Verification items for the finished model (mm, model axes). Coordinates: 2 decimals unless noted, no trailing zeros. Order: outer loops, then holes, each group sorted by start corner. A loop starts at its lowest first (then second) coordinate and runs counter-clockwise, first axis right, second up.
Q1. Depth check by flat-ended pin: P1, Ø6.5, axis at x = -5, z = -42.5, coming from the -Y side; P2, Ø3.5, axis at x = -5, z = -30, coming from the +Y side. Enter the tip coordinate at first touch or a pass-through.
Q2. Cross-section at A-A, the plane z = -42.5. Record the boundary of the cut face in (x, y).
Q3. Thickness scan on line 1 (Z direction, x = -5, y = 0.6); line 2 (X direction, y = 2.8, z = -16); line 3 (X direction, y = 2.6, z = -31). Record the ranges inside material, lowest first.
Q4. Draft check along X on faces 1 (the flat face through (-25, 0, -30)), 2 (the cylindrical face through (-4.74, 1.479, -19.483)), 3 (the flat face through (0, 1, -30)). Enter one of: pulls with the +X half, pulls with the -X half, needs draft (parallel to the pull), parting line crosses it, or undercut.
Autodesk Inventor part; units mm, degrees
ref_plane "YZ Plane" through (0, 0, 0) normal (1, 0, 0) x (0, 1, 0)
ref_plane "XZ Plane" through (0, 0, 0) normal (0, 1, 0) x (-1, 0, 0)
ref_plane "XY Plane" through (0, 0, 0) normal (0, 0, 1) x (1, 0, 0)
sketch "Sketch1" plane through (0, 0, 0) normal (0, 1, 0) x (-1, 0, 0)
  line L0 (0, 0) -> (50, 0)
  line L1 (50, 0) -> (50, -60)
  line L2 (50, -60) -> (0, -60)
  line L3 (0, -60) -> (0, 0)
  circle A0 centre (5, -30) radius 2
  circle A1 centre (5, -42.5) radius 2
  circle A2 centre (5, -17.5) radius 2
  dimension "d0" = 50
  dimension "d1" = 60
  dimension "d2" = 4
  dimension "d3" = 4
  dimension "d4" = 4
extrude "Extrusion1" add sketch "Sketch1" along normal blind 3
properties part number "dc clamps"
Check values:
1. P1: stops at y = 0
1. P2: passes through
2. outline: (-50, 0) - (-7, 0) - (-7, 3) - (-50, 3) - close; (-3, 0) - (0, 0) - (0, 3) - (-3, 3) - close
3. line 1: z = -60 to -44.5, -40.5 to -32, -28 to -19.5, -15.5 to 0
3. line 2: x = -50 to -6.32, -3.68 to 0
3. line 3: x = -50 to -6.73, -3.27 to 0
4. face 1: needs draft
4. face 2: undercut
4. face 3: pulls with the +X half
